from build123d import *

# Parameters (mm, degrees)
SKETCH1_W               = 100
SKETCH1_H               = 40
BOSS_EXTRUDE1_DEPTH     = 3
SKETCH2_W               = 15
SKETCH2_H               = 15
BOSS_EXTRUDE2_DEPTH     = 3
SKETCH3_R               = 1
BOSS_EXTRUDE3_DEPTH     = 15
CUT_EXTRUDE1_REACH      = 68.65
SKETCH4_W               = 4.7
SKETCH4_H               = 12.5
MIRROR2_COPY_1_SKETCH_R = 1
MIRROR2_COPY_1_DEPTH    = 15
MIRROR2_COPY_2_REACH    = 68.65
MIRROR2_COPY_2_SKETCH_W = 4.7
MIRROR2_COPY_2_SKETCH_H = 12.5


with BuildPart() as part:
    # Sketch1 → Boss-Extrude1 (new body)
    with BuildSketch(Plane.XY):
        Rectangle(SKETCH1_W, SKETCH1_H)
    extrude(amount=BOSS_EXTRUDE1_DEPTH)

    # Sketch2 → Boss-Extrude2 (add)
    with BuildSketch(Plane.XY.offset(3)):
        with Locations((-42.5, 12.5)):
            Rectangle(SKETCH2_W, SKETCH2_H)
        with Locations((-42.5, -12.5)):
            Rectangle(SKETCH2_W, SKETCH2_H)
        with Locations((42.5, -12.5)):
            Rectangle(SKETCH2_W, SKETCH2_H)
        with Locations((42.5, 12.5)):
            Rectangle(SKETCH2_W, SKETCH2_H)
    extrude(amount=BOSS_EXTRUDE2_DEPTH)

    # Sketch3 → Boss-Extrude3 (add)
    with BuildSketch(Plane.ZY.offset(50)):
        with BuildLine():
            Line((6, 5), (14.951381156, 7.715285511))
            ThreePointArc((14.951381156, 7.715285511), (18.5, 12.5), (14.951381156, 17.284714489))
            Line((14.951381156, 17.284714489), (6, 20))
            Line((6, 20), (6, 5))
        make_face()
        with Locations(Location((13.5, 12.5, 0), (0, 0, 270))):
            Circle(SKETCH3_R, mode=Mode.SUBTRACT)
    boss_extrude3 = extrude(amount=-BOSS_EXTRUDE3_DEPTH)

    # Sketch4 → Cut-Extrude1 (cut, up to next)
    with BuildSketch(Plane(origin=(0, 20, 0), x_dir=(1, 0, 0), z_dir=(0, 1, 0)), mode=Mode.PRIVATE) as cut_extrude1_sk1:
        with Locations((-37.35, -12.25)):
            Rectangle(SKETCH4_W, SKETCH4_H)
    cut_extrude1_tool1 = extrude(cut_extrude1_sk1.sketch, amount=-CUT_EXTRUDE1_REACH, mode=Mode.PRIVATE) & part.part
    # Sketch4 → Cut-Extrude1 (cut, up to next)
    with BuildSketch(Plane(origin=(0, 20, 0), x_dir=(1, 0, 0), z_dir=(0, 1, 0)), mode=Mode.PRIVATE) as cut_extrude1_sk2:
        with Locations((-47.65, -12.25)):
            Rectangle(SKETCH4_W, SKETCH4_H)
    cut_extrude1_tool2 = extrude(cut_extrude1_sk2.sketch, amount=-CUT_EXTRUDE1_REACH, mode=Mode.PRIVATE) & part.part
    cut_extrude1_1 = cut_extrude1_tool1.solids().sort_by_distance((-37.35, 20, 12.25))[0]
    add(cut_extrude1_1, mode=Mode.SUBTRACT)
    cut_extrude1_2 = cut_extrude1_tool2.solids().sort_by_distance((-47.65, 20, 12.25))[0]
    add(cut_extrude1_2, mode=Mode.SUBTRACT)
    cut_extrude1 = cut_extrude1_1 + cut_extrude1_2  # Cut-Extrude1 as one shape, for the pattern or mirror that repeats it

    # Mirror1: Boss-Extrude3, Cut-Extrude1 across plane
    add(boss_extrude3.mirror(Plane.ZX))
    add(cut_extrude1.mirror(Plane.ZX), mode=Mode.SUBTRACT)

    # Mirror2: Boss-Extrude3, Cut-Extrude1 across plane
    add(boss_extrude3.mirror(Plane(origin=(0, 0, 0), x_dir=(0, 0, 1), z_dir=(1, 0, 0))))
    add(cut_extrude1.mirror(Plane(origin=(0, 0, 0), x_dir=(0, 0, 1), z_dir=(1, 0, 0))), mode=Mode.SUBTRACT)

    # Mirror2 copy 1 sketch → Mirror2 copy 1 (add)
    with BuildSketch(Plane(origin=(50, 0, 0), x_dir=(0, 0, 1), z_dir=(1, 0, 0))):
        with BuildLine():
            Line((6, 5), (14.951381156, 7.715285511))
            ThreePointArc((14.951381156, 7.715285511), (18.5, 12.5), (14.951381156, 17.284714489))
            Line((14.951381156, 17.284714489), (6, 20))
            Line((6, 20), (6, 5))
        make_face()
        with Locations(Location((13.5, 12.5, 0), (0, 0, 270))):
            Circle(MIRROR2_COPY_1_SKETCH_R, mode=Mode.SUBTRACT)
    extrude(amount=-MIRROR2_COPY_1_DEPTH)

    # Mirror2 copy 2 sketch → Mirror2 copy 2 (cut, up to next)
    with BuildSketch(Plane(origin=(0, -20, 0), x_dir=(-1, 0, 0), z_dir=(0, -1, 0)), mode=Mode.PRIVATE) as mirror2_copy_2_sk1:
        with Locations((-37.35, -12.25)):
            Rectangle(MIRROR2_COPY_2_SKETCH_W, MIRROR2_COPY_2_SKETCH_H)
    mirror2_copy_2_tool1 = extrude(mirror2_copy_2_sk1.sketch, amount=-MIRROR2_COPY_2_REACH, mode=Mode.PRIVATE) & part.part
    # Mirror2 copy 2 sketch → Mirror2 copy 2 (cut, up to next)
    with BuildSketch(Plane(origin=(0, -20, 0), x_dir=(-1, 0, 0), z_dir=(0, -1, 0)), mode=Mode.PRIVATE) as mirror2_copy_2_sk2:
        with Locations((-47.65, -12.25)):
            Rectangle(MIRROR2_COPY_2_SKETCH_W, MIRROR2_COPY_2_SKETCH_H)
    mirror2_copy_2_tool2 = extrude(mirror2_copy_2_sk2.sketch, amount=-MIRROR2_COPY_2_REACH, mode=Mode.PRIVATE) & part.part
    add(mirror2_copy_2_tool1.solids().sort_by_distance((37.35, -20, 12.25))[0], mode=Mode.SUBTRACT)
    add(mirror2_copy_2_tool2.solids().sort_by_distance((47.65, -20, 12.25))[0], mode=Mode.SUBTRACT)


solid = part.part
Work out the finished part from the listing and answer in its coordinate system (mm). A direction names the side the tool comes from. Coordinates: 2 decimals unless noted, no trailing zeros. Loops run counter-clockwise (first coordinate to the right, second up) from the corner with the lowest first, then second, coordinate; pieces in that order, holes last. Notation, with made-up numbers: M -32,65.5 L 14,65.5 A12 cw 14,86.5 Z; hole C 47,38.25 d11. An arc over 180 degrees is marked long. Answer in a Markdown table with one row per item. Add a question column.
1. The mould has two halves that part along Y. Classify faces 4 (the flat face through (-1, 20, 2)), 5 (the flat face through (37, 13, 6)), 6 (the flat face through (42, -5, 4)), 7 (the cylindrical face through (42.5, -12.4, 18.5)): pulls with the +Y half, pulls with the -Y half, needs draft (parallel to the pull), parting line crosses it, or undercut.
2. Find section D-D, the plane y = 2.5. Write down the section's boundary in (x, z).
3. Find section C-C, the plane z = 13.5. State how many separate pieces and enclosed holes the cut face has, then the cut area to 3 significant figures.
4. Flat-ended cylindrical pins translate along their axes: P1, Ø20, axis at x = -20, y = 3, coming from the +Z side; P2, Ø1.4, axis at x = -47, y = -15.5, coming from the +Z side; P3, Ø10, axis at y = 11.5, z = 14.5, coming from the -X side. Find the tip coordinate at first contact, or state that the pin passes through.
5. Find section B-B, the plane x = -41. Write down the section's boundary in (y, z), then the cut area to 3 significant figures.
6. A tool of negligible diameter and unlimited length cuts with its end or side. For faces 1 (the flat face through (45.3, 13, 11)), 2 (the flat face through (-45.3, -13, 11)), 3 (the flat face through (39.7, 13, 11)), from which of +Z, -Z, +X, -X, +Y, -Y can it reach the whole face along a straight path? Write none if from no direction.
7. Consider L1, parallel to X at y = 15.5, z = 9; L2, parallel to Z at x = -42.05, y = 12.5; L3, parallel to Y at x = 44, z = 14. Determine where each line is inside the solid, lowest interval first.
8. Find section A-A, the plane y = 12.5. Write down the section's boundary in (x, z).
Reported:
| question | item | result |
|---|---|---|
| 1 | face 4 | pulls with the +Y half |
| 1 | face 5 | needs draft |
| 1 | face 6 | undercut |
| 1 | face 7 | undercut |
| 2 | outline | M -50,0 L 50,0 L 50,3 L -50,3 Z |
| 3 | separate pieces | 8 |
| 3 | enclosed holes | 0 |
| 3 | area | 189 mm^2 |
| 4 | P1 | stops at z = 3 |
| 4 | P2 | stops at z = 6 |
| 4 | P3 | stops at x = -45.3 |
| 5 | outline | M -20,0 L 20,0 L 20,6 L 17.28,14.95 A5 ccw 7.72,14.95 L 5,6 L 5,3 L -5,3 L -5,6 L -7.72,14.95 A5 ccw -17.28,14.95 L -20,6 Z; hole C -12.5,13.5 d2; hole C 12.5,13.5 d2 |
| 5 | area | 474 mm^2 |
| 6 | face 1 | +Z, +X, +Y, -Y |
| 6 | face 2 | +Z, -X, +Y, -Y |
| 6 | face 3 | +Z, +Y, -Y |
| 7 | L1 | x = -45.3 to -39.7, 39.7 to 45.3 |
| 7 | L2 | z = 0 to 12.5, 14.5 to 18.5 |
| 7 | L3 | y = -17.57 to -13.37, -11.63 to -7.43, 7.43 to 11.63, 13.37 to 17.57 |
| 8 | outline | M -50,0 L 50,0 L 50,6 L 45.3,6 L 45.3,12.5 L 39.7,12.5 L 39.7,6 L 35,6 L 35,3 L -35,3 L -35,6 L -39.7,6 L -39.7,12.5 L -45.3,12.5 L -45.3,6 L -50,6 Z; M -45.3,14.5 L -39.7,14.5 L -39.7,18.5 L -45.3,18.5 Z; M 39.7,14.5 L 45.3,14.5 L 45.3,18.5 L 39.7,18.5 Z |
